Check sheet for the modelled part. Datum: model origin and axes. Units: mm. A direction names the side the tool comes from. Round coordinates to 2 decimals unless told otherwise and drop trailing zeros. Loops run counter-clockwise (first coordinate to the right, second up) from the corner with the lowest first, then second, coordinate; pieces in that order, holes last. Notation, with made-up numbers: (2.5, -21.5) - (21.5, -21.5) arc R22 ccw to (21.5, 7.5) - close; hole circle Ø2 at (-17, 51.25). An arc over 180 degrees is marked (long way). Return JSON: item names as keys, results as strings.
from build123d import *

# Parameters (mm, degrees)
F0_W     = 46
F0_H     = 46
F1_DEPTH = 725
F3_W     = 46
F3_H     = 46
F4_DEPTH = 25


with BuildPart() as f1:
    # F0 (on Right) → F1 (new body, symmetric)
    with BuildSketch(Plane.YZ):
        with BuildLine():
            ThreePointArc((-175, 422.46), (-175.743949, 424.256051), (-177.54, 425))
            Line((-177.54, 425), (-222.46, 425))
            ThreePointArc((-222.46, 425), (-224.256051, 424.256051), (-225, 422.46))
            Line((-225, 422.46), (-225, 377.54))
            ThreePointArc((-225, 377.54), (-224.256051, 375.743949), (-222.46, 375))
            Line((-222.46, 375), (-177.54, 375))
            ThreePointArc((-177.54, 375), (-175.743949, 375.743949), (-175, 377.54))
            Line((-175, 377.54), (-175, 422.46))
        make_face()
        with Locations((-200, 400)):
            Rectangle(F0_W, F0_H, mode=Mode.SUBTRACT)
    extrude(amount=F1_DEPTH, both=True)

    # F3 (on offset) → F4 (join, symmetric)
    with BuildSketch(Plane.XY.offset(400)):
        with BuildLine():
            Line((727.54, -225), (772.46, -225))
            ThreePointArc((772.46, -225), (774.256051, -224.256051), (775, -222.46))
            Line((775, -222.46), (775, -177.54))
            ThreePointArc((775, -177.54), (774.256051, -175.743949), (772.46, -175))
            Line((772.46, -175), (727.54, -175))
            ThreePointArc((727.54, -175), (725.743949, -175.743949), (725, -177.54))
            Line((725, -177.54), (725, -222.46))
            ThreePointArc((725, -222.46), (725.743949, -224.256051), (727.54, -225))
        make_face()
        with Locations((750, -200)):
            Rectangle(F3_W, F3_H, mode=Mode.SUBTRACT)
        with BuildLine():
            ThreePointArc((-775, -222.46), (-774.256051, -224.256051), (-772.46, -225))
            Line((-772.46, -225), (-727.54, -225))
            ThreePointArc((-727.54, -225), (-725.743949, -224.256051), (-725, -222.46))
            Line((-725, -222.46), (-725, -177.54))
            ThreePointArc((-725, -177.54), (-725.743949, -175.743949), (-727.54, -175))
            Line((-727.54, -175), (-772.46, -175))
            ThreePointArc((-772.46, -175), (-774.256051, -175.743949), (-775, -177.54))
            Line((-775, -177.54), (-775, -222.46))
        make_face()
        with Locations((-750, -200)):
            Rectangle(F3_W, F3_H, mode=Mode.SUBTRACT)
    extrude(amount=F4_DEPTH, both=True)


solid = f1.part
Q1. Sectioned sample at C-C (x = 311). Enter the section's corners in (y, z).
Answer key:
{"outline": "(-225, 377.54) arc R2.54 ccw to (-222.46, 375) - (-177.54, 375) arc R2.54 ccw to (-175, 377.54) - (-175, 422.46) arc R2.54 ccw to (-177.54, 425) - (-222.46, 425) arc R2.54 ccw to (-225, 422.46) - close; hole (-223, 377) - (-177, 377) - (-177, 423) - (-223, 423) - close"}
Q2. Tool access check on faces 1 (the face through (-750, -223, 400)), 2 (the face through (10, -177, 400)), 3 (the face through (-775, -200, 400)). Record the directions out of +Z, -Z, +X, -X, +Y, -Y that give a thin tool (end or side, any length) a straight path to the whole face; none if there is none.
Answer key:
{"face 1": "+Z, -Z", "face 2": "none", "face 3": "+Z, -Z, -X, +Y, -Y"}
Q3. Draft check along Z on faces 4 (the face through (750, -177, 400)), 5 (the face through (-11, -205, 375)), 6 (the face through (10, -200, 423)). Enter one of: released by +Z, released by -Z, zero draft, split by the parting line, or undercut.
Answer key:
{"face 4": "zero draft", "face 5": "released by -Z", "face 6": "undercut"}
Q4. Depth check by flat-ended pin: P1, Ø0.8, axis at y = -176, z = 405.5, coming from the +X side; P2, Ø2, axis at y = -176, z = 390, coming from the -X side. Enter the tip coordinate at first touch or a pass-through.
Answer key:
{"P1": "stops at x = 774.73", "P2": "stops at x = -774.94"}
Q5. Sectioned sample at B-B (y = -211.5). Enter the section's corners in (x, z).
Answer key:
{"outline": "(-775, 375) - (-773, 375) - (-773, 425) - (-775, 425) - close; (-727, 375) - (727, 375) - (727, 425) - (-727, 425) - close; (773, 375) - (775, 375) - (775, 425) - (773, 425) - close; hole (-725, 377) - (725, 377) - (725, 423) - (-725, 423) - close"}
Q6. Sectioned sample at A-A (z = 404.5). State how many separate pieces and enclosed holes the cut face has, plus the area to 3 significant figures.
Answer key:
{"separate pieces": "4", "enclosed holes": "2", "area": "6,560 mm²"}
Q7. Scan lines: probe 1 along X at (y, z) = (-188.5, 405); probe 2 along Y at (x, z) = (-169, 392); probe 3 along Z at (x, y) = (115, -218.5). Record each from-to range of solid material in increasing order. Write a range as [from, to].
Answer key:
{"probe 1": "x = [-775, -773], [-727, -725], [725, 727], [773, 775]", "probe 2": "y = [-225, -223], [-177, -175]", "probe 3": "z = [375, 377], [423, 425]"}
